```python
from build123d import *
from build123d.topology import SkipClean

# Parameters (mm, degrees)
SKETCH3_R           = 55
BOSS_EXTRUDE2_DEPTH = 25
SKETCH4_R           = 50
CUT_EXTRUDE1_DEPTH  = 15
CUT_EXTRUDE2_START  = -15
CUT_EXTRUDE2_DEPTH  = 15
BOSS_EXTRUDE3_DEPTH = 10
BOSS_EXTRUDE4_DEPTH = 10
BOSS_EXTRUDE5_DEPTH = 15
CUT_EXTRUDE4_START  = -15
CUT_EXTRUDE4_DEPTH  = 15
SKETCH11_R          = 2.5
CUT_EXTRUDE7_DEPTH  = 25
SKETCH12_R          = 2.5
CUT_EXTRUDE9_DEPTH  = 10
CUT_EXTRUDE12_DEPTH = 5
SKETCH14_R          = 5
CUT_EXTRUDE13_DEPTH = 10
BOSS_EXTRUDE6_START = 10
BOSS_EXTRUDE6_DEPTH = 10


with BuildPart() as part:
    # Sketch3 → Boss-Extrude2 (new body)
    with BuildSketch(Plane.XY):
        Circle(SKETCH3_R)
    extrude(amount=BOSS_EXTRUDE2_DEPTH)

    # Sketch4 → Cut-Extrude1 (cut)
    with BuildSketch(Plane(origin=(0, 0, 0), x_dir=(-1, 0, 0), z_dir=(0, 0, -1))):
        Circle(SKETCH4_R)
    extrude(amount=-CUT_EXTRUDE1_DEPTH, mode=Mode.SUBTRACT)

    # Sketch5 → Cut-Extrude2 (cut)
    with BuildSketch(Plane.XY.offset(25).offset(CUT_EXTRUDE2_START)):
        with BuildLine():
            ThreePointArc((-52.915026221, 15), (-46.143782777, 0), (-52.915026221, -15))
            ThreePointArc((-52.915026221, -15), (-55, 0), (-52.915026221, 15))
        make_face()
    extrude(amount=CUT_EXTRUDE2_DEPTH, mode=Mode.SUBTRACT)

    # Sketch6 → Boss-Extrude3 (add)
    with BuildSketch(Plane.XY.offset(25)):
        with BuildLine():
            Line((-35, 15), (-20, 15))
            ThreePointArc((-20, 15), (-11.180339887, 22.360679775), (0, 25))
            Line((0, 25), (0, 40))
            ThreePointArc((0, 40), (-21.505813168, 33.108138435), (-35, 15))
        make_face()
    extrude(amount=BOSS_EXTRUDE3_DEPTH)

    # Sketch7 → Boss-Extrude4 (add)
    with BuildSketch(Plane.XY.offset(25)):
        with BuildLine():
            Line((-35, -15), (-20, -15))
            ThreePointArc((-20, -15), (-11.180339887, -22.360679775), (0, -25))
            Line((0, -25), (0, -40))
            ThreePointArc((0, -40), (-21.505813168, -33.108138435), (-35, -15))
        make_face()
    extrude(amount=BOSS_EXTRUDE4_DEPTH)

    # Sketch8 → Boss-Extrude5 (add)
    with SkipClean():  # the faces are left unmerged after this step: merging them gives an invalid solid
        with BuildSketch(Plane.XY.offset(25)):
            with BuildLine():
                Line((0, -40), (0, -25))
                ThreePointArc((0, -25), (25, 0), (0, 25))
                Line((0, 25), (0, 40))
                ThreePointArc((0, 40), (40, 0), (0, -40))
            make_face()
        extrude(amount=BOSS_EXTRUDE5_DEPTH)

    # Sketch9 → Cut-Extrude4 (cut)
    with SkipClean():  # the faces are left unmerged after this step: merging them gives an invalid solid
        with BuildSketch(Plane.XY.offset(40).offset(CUT_EXTRUDE4_START)):
            with BuildLine():
                Line((19.014552984, -29.474791897), (22.456700597, -33.101308106))
                ThreePointArc((22.456700597, -33.101308106), (27.537180907, -29.012129665), (31.885642738, -24.151724311))
                Line((31.885642738, -24.151724311), (28.443495125, -20.525208103))
                ThreePointArc((28.443495125, -20.525208103), (19.254232157, -20.285528929), (19.014552984, -29.474791897))
            make_face()
            with BuildLine():
                Line((22.456700597, 33.101308106), (19.014552984, 29.474791897))
                ThreePointArc((19.014552984, 29.474791897), (19.254232157, 20.285528929), (28.443495125, 20.525208103))
                Line((28.443495125, 20.525208103), (31.885642738, 24.151724311))
                ThreePointArc((31.885642738, 24.151724311), (27.537180907, 29.012129665), (22.456700597, 33.101308106))
            make_face()
        extrude(amount=CUT_EXTRUDE4_DEPTH, mode=Mode.SUBTRACT)

    # Sketch11 → Cut-Extrude7 (cut)
    with SkipClean():  # the faces are left unmerged after this step: merging them gives an invalid solid
        with BuildSketch(Plane.XY.offset(25)):
            with Locations((23.729024054, -25)):
                Circle(SKETCH11_R)
            with Locations((23.729024054, 25)):
                Circle(SKETCH11_R)
        extrude(amount=-CUT_EXTRUDE7_DEPTH, mode=Mode.SUBTRACT)

    # Sketch12 → Cut-Extrude9 (cut)
    with SkipClean():  # the faces are left unmerged after this step: merging them gives an invalid solid
        with BuildSketch(Plane.XY.offset(25)):
            with Locations((15, 0)):
                Circle(SKETCH12_R)
        extrude(amount=-CUT_EXTRUDE9_DEPTH, mode=Mode.SUBTRACT)

    # Sketch13 → Cut-Extrude12 (cut)
    with SkipClean():  # the faces are left unmerged after this step: merging them gives an invalid solid
        with BuildSketch(Plane.XY.offset(25)):
            with BuildLine():
                Line((-25, 10), (0, 10))
                ThreePointArc((0, 10), (10, 0), (0, -10))
                Line((0, -10), (-25, -10))
                ThreePointArc((-25, -10), (-35, 0), (-25, 10))
            make_face()
        extrude(amount=-CUT_EXTRUDE12_DEPTH, mode=Mode.SUBTRACT)

    # Sketch14 → Cut-Extrude13 (cut)
    with SkipClean():  # the faces are left unmerged after this step: merging them gives an invalid solid
        with BuildSketch(Plane.XY.offset(20)):
            with Locations((-25, 0)):
                Circle(SKETCH14_R)
            Circle(SKETCH14_R)
        extrude(amount=-CUT_EXTRUDE13_DEPTH, mode=Mode.SUBTRACT)

    # Sketch15 → Boss-Extrude6 (add)
    with SkipClean():  # the faces are left unmerged after this step: merging them gives an invalid solid
        with BuildSketch(Plane.XY.offset(20).offset(BOSS_EXTRUDE6_START)):
            with BuildLine():
                Line((0, 5), (0, 10))
                ThreePointArc((0, 10), (10, 0), (0, -10))
                Line((0, -10), (0, -5))
                ThreePointArc((0, -5), (5, 0), (0, 5))
            make_face()
        extrude(amount=-BOSS_EXTRUDE6_DEPTH)


solid = part.part
```
Geometry check sheet. Reference: the model listing, model coordinates, mm. A direction names the side the tool comes from. Give positions to 0.01 mm unless a question says otherwise; leave off trailing zeros. Write each loop counter-clockwise with the first axis right and the second up, starting at its lowest first coordinate (ties: lowest second). Pieces come first, ordered by that corner, then holes.
1) Release check for a two-part mould opening along X. For faces 1 (the cylindrical face through (19.36, -20.19, 32.39)), 2 (the cylindrical face through (50.806, -21.065, 12.325)), 3 (the flat face through (-28, -15, 30)) record: pulls with the +X half, pulls with the -X half, needs draft (parallel to the pull), parting line crosses it, or undercut.
2) Access from +Z, -Z, +X, -X, +Y, -Y to the whole of each face (thin tool, end or side, straight path). Record for faces 4 (the cylindrical face through (-21.244, -33.294, 29.93)), 5 (the cylindrical face through (-35, 0, 23)), 6 (the cylindrical face through (11.906, -38.187, 32.395)), 7 (the flat face through (30.14, 22.31, 32.39)), 8 (the cylindrical face through (-21.244, 33.294, 29.93)).
3) Section check D-D, the plane x = 14. Record the boundary of the cut face in (y, z).
4) Gauge pin test, flat ends, axial feed: pin 1 (20 mm diameter, centred on x = -15.5, y = -23, fed in from +Z); pin 2 (12 mm diameter, centred on x = 44, y = -19.5, fed in from +Z); pin 3 (10 mm diameter, centred on x = -13, y = 2.5, fed in from +Z); pin 4 (4 mm diameter, centred on x = 23.73, y = -25, fed in from +Z). Record the tip position at first contact, or that the pin passes through.
5) Section check C-C, the plane x = -33.5. Record the boundary of the cut face in (y, z).
6) Material ranges on L1, parallel to Y at x = 0, z = 11; L2, parallel to Z at x = 13, y = 9; L3, parallel to Z at x = 47, y = 27, recorded low to high.
7) Section check B-B, the plane z = 33. Record the boundary of the cut face in (x, y).
8) Section check A-A, the plane y = 0. State how many separate pieces and enclosed holes the cut face has, and give its area (3 significant figures).
Computed:
1. face 1: undercut
1. face 2: parting line crosses it
1. face 3: needs draft
2. face 4: +Z, -X, -Y
2. face 5: +Z
2. face 6: +Z, +X, -Y
2. face 7: +Z, +Y
2. face 8: +Z, -X, +Y
3. outline: (-53.19, 0) - (-48, 0) - (-48, 15) - (-2.29, 15) - (-2.29, 25) - (-20.71, 25) - (-20.71, 40) - (-37.47, 40) - (-37.47, 25) - (-53.19, 25) - close; (2.29, 15) - (48, 15) - (48, 0) - (53.19, 0) - (53.19, 25) - (37.47, 25) - (37.47, 40) - (20.71, 40) - (20.71, 25) - (2.29, 25) - close
4. pin 1: stops at z = 35
4. pin 2: stops at z = 25
4. pin 3: stops at z = 20
4. pin 4: passes through
5. outline: (-43.62, 0) - (-37.12, 0) - (-37.12, 15) - (37.12, 15) - (37.12, 0) - (43.62, 0) - (43.62, 25) - (18.71, 25) - (18.71, 35) - (15, 35) - (15, 25) - (5.27, 25) - (5.27, 20) - (-5.27, 20) - (-5.27, 25) - (-15, 25) - (-15, 35) - (-18.71, 35) - (-18.71, 25) - (-43.62, 25) - close
6. L1: y = -55 to -50, 50 to 55
6. L2: z = 15 to 25
6. L3: z = 0 to 25
7. outline: (-35, -15) arc R37 ccw to (0, -40) arc R40 ccw to (22.46, -33.1) - (19.01, -29.47) arc R6.5 cw to (28.44, -20.53) - (31.89, -24.15) arc R40 ccw to (31.89, 24.15) - (28.44, 20.53) arc R6.5 cw to (19.01, 29.47) - (22.46, 33.1) arc R40 ccw to (0, 40) arc R37 ccw to (-35, 15) - (-20, 15) arc R25 cw (long way) to (-20, -15) - close
8. separate pieces: 5
8. enclosed holes: 0
8. area: 1,040 mm2
